from build123d import *

# Parameters (mm, degrees)
F0_W     = 6
F0_H     = 7.4
F2_R     = 2.5
F3_DEPTH = 9


with BuildPart() as f1:
    # F0 (on Front) → F1 (revolve)
    with BuildSketch(Plane.XZ):
        Polygon((0, 11.687311), (-9, 11.687311), (-8.2, 10.887311), (-6, 10.887311), (0, 10.887311), align=None)
        with Locations((-3, 7.187311)):
            Rectangle(F0_W, F0_H)
        Polygon((0, 2.687311), (0, 3.487311), (-6, 3.487311), (-8.2, 3.487311), (-9, 2.687311), align=None)
    revolve(axis=Axis((0, 0, 3.487311), (0, 0, 1)))

    # F2 (on face) → F3 (cut, through all)
    with BuildSketch(Plane.XY.offset(11.687311)):
        Circle(F2_R)
    extrude(amount=-F3_DEPTH, mode=Mode.SUBTRACT)


solid = f1.part
The listing builds one solid part. Answer for the finished solid, in the listing's coordinates (mm). A direction names the side the tool comes from. Give positions to 0.01 mm unless a question says otherwise; leave off trailing zeros. Write each loop counter-clockwise with the first axis right and the second up, starting at its lowest first coordinate (ties: lowest second). Pieces come first, ordered by that corner, then holes. Notation, with made-up numbers: (8.5, 44.25) - (29.5, 44.25) arc R31 cw to (29.5, 77.25) - close; hole circle Ø8 at (-19, 53.25). An arc over 180 degrees is marked (long way). Use a Markdown table: item, result.
1. Section A-A on y = 0 is taken. Write down the section's boundary in (x, z).
Values follow:
| item | result |
|---|---|
| outline | (-9, 2.69) - (-2.5, 2.69) - (-2.5, 11.69) - (-9, 11.69) - (-8.2, 10.89) - (-6, 10.89) - (-6, 3.49) - (-8.2, 3.49) - close; (2.5, 2.69) - (9, 2.69) - (8.2, 3.49) - (6, 3.49) - (6, 10.89) - (8.2, 10.89) - (9, 11.69) - (2.5, 11.69) - close |
2. Each of these flat-tipped pins is pushed along its axis until it touches: P1, Ø1.5, axis at x = 5.5, z = 7.5, coming from the -Y side; P2, Ø5, axis at y = 6.5, z = 6.5, coming from the +X side; P3, Ø1, axis at x = -3.5, z = 6.5, coming from the -Y side. Where does it stop, or does it pass through?
Values follow:
| item | result |
|---|---|
| P1 | stops at y = -3.67 |
| P2 | stops at x = 4.47 |
| P3 | stops at y = -5.2 |
3. A tool of negligible diameter and unlimited length cuts with its end or side. For faces 4 (the flat face through (-4, 5, 10.887)), 5 (the cylindrical face through (-0.54, -2.44, 7.25)), from which of +Z, -Z, +X, -X, +Y, -Y can it reach the whole face along a straight path? Write none if from no direction.
Values follow:
| item | result |
|---|---|
| face 4 | none |
| face 5 | +Z, -Z |
4. For a pull along Z with two mould halves and no side action, classify faces 1 (the flat face through (2, 2, 11.687)), 2 (the flat face through (4, 5, 3.487)), 3 (the flat face through (-2, 2, 2.687)) as released by +Z, released by -Z, zero draft, split by the parting line, or undercut.
Values follow:
| item | result |
|---|---|
| face 1 | released by +Z |
| face 2 | undercut |
| face 3 | released by -Z |
5. Find the intervals of material crossed by probe 1 along Y at (x, z) = (0, 4.5); probe 2 along Z at (x, y) = (-6.75, -1.5); probe 3 along X at (y, z) = (1, 9.75), in increasing order. Write a range as from..to.
Values follow:
| item | result |
|---|---|
| probe 1 | y = -6..-2.5, 2.5..6 |
| probe 2 | z = 2.69..3.49, 10.89..11.69 |
| probe 3 | x = -5.92..-2.29, 2.29..5.92 |
6. Section C-C on z = 5.75 is taken. Write down the section's boundary in (x, y).
Values follow:
| item | result |
|---|---|
| outline | circle Ø12 at (0, 0); hole circle Ø5 at (0, 0) |
